Part model, mm, in its own coordinate system. Coordinates: 2 decimals unless noted, no trailing zeros. Loops run counter-clockwise (first coordinate to the right, second up) from the corner with the lowest first, then second, coordinate; pieces in that order, holes last. Notation, with made-up numbers: (59, 30) - (89, 30) arc R21 ccw to (89, 53) - close; hole circle Ø10 at (56, -19). An arc over 180 degrees is marked (long way). Use a Markdown table: item, result. Add a question column.
1. Band-saw the part on B-B, the plane x = 35.5. Give the cut face in (y, z), plus the area to 3 significant figures.
2. Band-saw the part on A-A, the plane z = 58.5. Give the cut face in (x, y), plus the area to 3 significant figures.
3. Wall check: probe 1 along Z at (x, y) = (-15, -30); probe 2 along Y at (x, z) = (6.5, 44). Give the ranges that are in metal, low to high. Write a range as [from, to].
4. Drop a flat-ended pin along its axis: pin 1 (2 mm diameter, centred on x = -40.5, z = 99, fed in from +Y). Give the stop position or say it passes through.
5. Band-saw the part on C-C, the plane z = 12. Give the cut face in (x, y), plus the area to 3 significant figures.
from build123d import *

# Parameters (mm, degrees)
SKETCH1_W           = 125
SKETCH1_H           = 68
BOSS_EXTRUDE1_DEPTH = 182.6
SKETCH2_W           = 172.6
SKETCH2_H           = 58
CUT_EXTRUDE1_DEPTH  = 126
SKETCH3_W           = 115
SKETCH3_H           = 58
CUT_EXTRUDE2_DEPTH  = 183.6
SKETCH4_W           = 115
SKETCH4_H           = 172.6
CUT_EXTRUDE3_DEPTH  = 63
SKETCH5_W           = 105
SKETCH5_H           = 20
CUT_EXTRUDE4_DEPTH  = 6


with BuildPart() as part:
    # Sketch1 → Boss-Extrude1 (new body)
    with BuildSketch(Plane.XY):
        Rectangle(SKETCH1_W, SKETCH1_H)
    extrude(amount=BOSS_EXTRUDE1_DEPTH)

    # Sketch2 → Cut-Extrude1 (cut, through all)
    with BuildSketch(Plane(origin=(62.5, 0, 0), x_dir=(0, 0, -1), z_dir=(1, 0, 0))):
        with Locations((-91.3, 0)):
            Rectangle(SKETCH2_W, SKETCH2_H)
    extrude(amount=-CUT_EXTRUDE1_DEPTH, mode=Mode.SUBTRACT)

    # Sketch3 → Cut-Extrude2 (cut, through all)
    with BuildSketch(Plane(origin=(0, 0, 0), x_dir=(-1, 0, 0), z_dir=(0, 0, -1))):
        Rectangle(SKETCH3_W, SKETCH3_H)
    extrude(amount=-CUT_EXTRUDE2_DEPTH, mode=Mode.SUBTRACT)

    # Sketch4 → Cut-Extrude3 (cut)
    with BuildSketch(Plane(origin=(0, 34, 0), x_dir=(1, 0, 0), z_dir=(0, 1, 0))):
        with Locations((0, -91.3)):
            Rectangle(SKETCH4_W, SKETCH4_H)
    extrude(amount=-CUT_EXTRUDE3_DEPTH, mode=Mode.SUBTRACT)

    # Sketch5 → Cut-Extrude4 (cut, through all)
    with BuildSketch(Plane(origin=(0, -29, 0), x_dir=(1, 0, 0), z_dir=(0, 1, 0))):
        with Locations((0, -15)):
            Rectangle(SKETCH5_W, SKETCH5_H)
    extrude(amount=-CUT_EXTRUDE4_DEPTH, mode=Mode.SUBTRACT)


solid = part.part
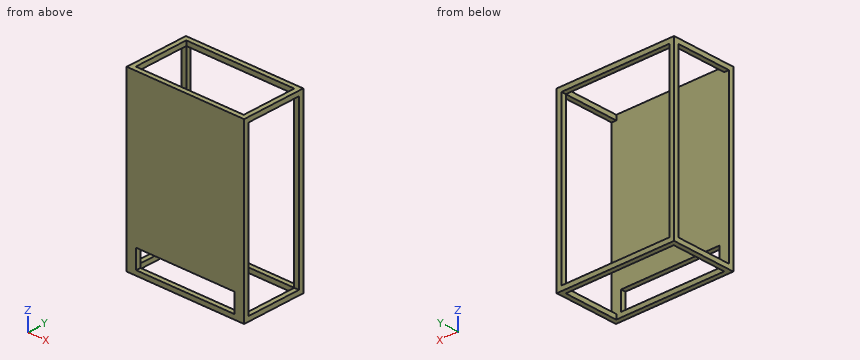
Geometry check:
| question | item | result |
|---|---|---|
| 1 | outline | (-34, 0) - (-29, 0) - (-29, 5) - (-34, 5) - close; (-34, 25) - (-29, 25) - (-29, 182.6) - (-34, 182.6) - close; (29, 0) - (34, 0) - (34, 5) - (29, 5) - close; (29, 177.6) - (34, 177.6) - (34, 182.6) - (29, 182.6) - close |
| 1 | area | 863 mm^2 |
| 2 | outline | (-62.5, -34) - (62.5, -34) - (62.5, -29) - (-62.5, -29) - close; (-62.5, 29) - (-57.5, 29) - (-57.5, 34) - (-62.5, 34) - close; (57.5, 29) - (62.5, 29) - (62.5, 34) - (57.5, 34) - close |
| 2 | area | 675 mm^2 |
| 3 | probe 1 | z = [0, 5], [25, 182.6] |
| 3 | probe 2 | y = [-34, -29] |
| 4 | pin 1 | stops at y = -29 |
| 5 | outline | (-62.5, -34) - (-52.5, -34) - (-52.5, -29) - (-62.5, -29) - close; (-62.5, 29) - (-57.5, 29) - (-57.5, 34) - (-62.5, 34) - close; (52.5, -34) - (62.5, -34) - (62.5, -29) - (52.5, -29) - close; (57.5, 29) - (62.5, 29) - (62.5, 34) - (57.5, 34) - close |
| 5 | area | 150 mm^2 |
